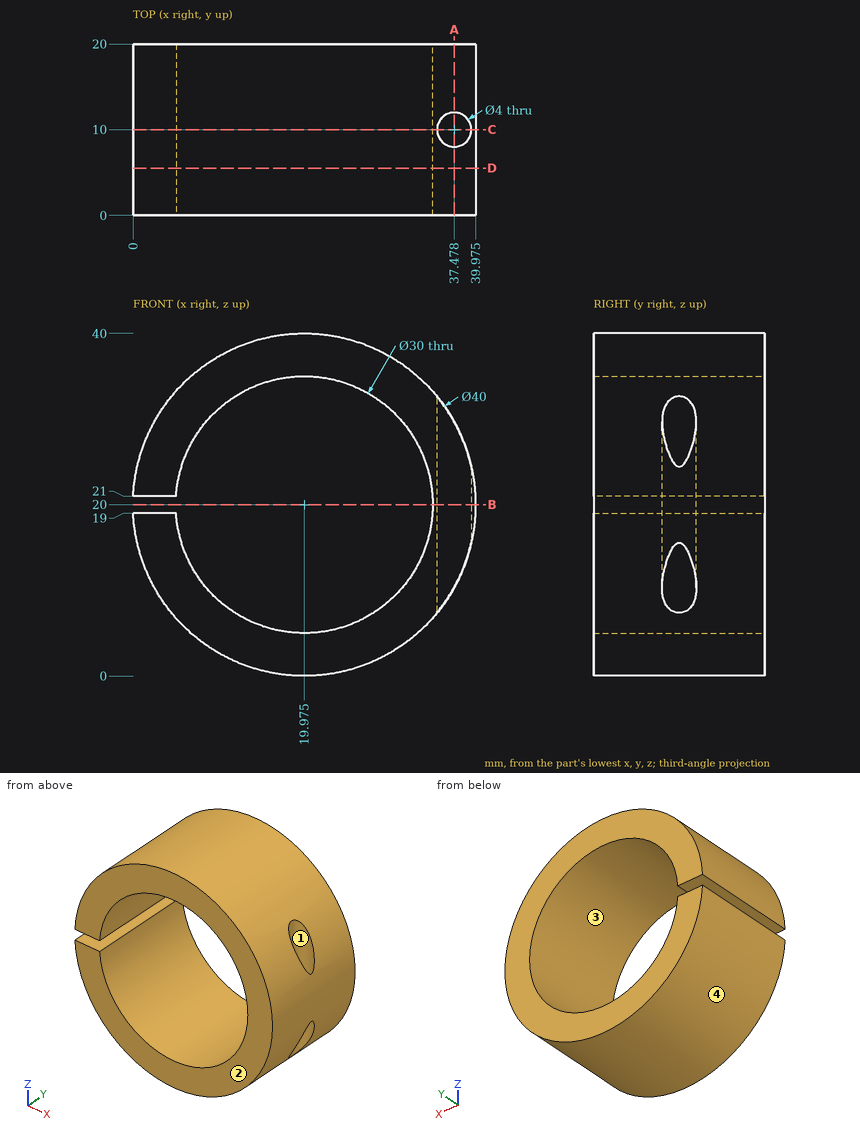
Input: dimensioned drawing with shaded views. Units: mm. Origin: part minimum x, y, z. Round coordinates to 2 decimals unless told otherwise and drop trailing zeros. Order: outer loops, then holes, each group sorted by start corner. A loop starts at its lowest first (then second) coordinate and runs counter-clockwise, first axis right, second up. Notation, with made-up numbers: (52, -31) - (76, -31) arc R32 ccw to (76, -3) - close; hole circle Ø11 at (38.5, 52). An arc over 180 degrees is marked (long way). Write item = value, one per line. Start each with the question number.
Q1. Cut plane B-B on z = 20. Return the cut outline in (x, y) (1 decimal).
Q2. Pin query (flat end, axial travel): pin 1 (6 mm diameter, centred on y = 6.5, z = 32, fed in from +X) (1 decimal); pin 2 (6 mm diameter, centred on y = 12.5, z = 30.5, fed in from -X) (1 decimal); pin 3 (8 mm diameter, centred on y = 2.5, z = 13.5, fed in from +X). Return the tip coordinate at first contact, or that it passes through.
Q3. Cut plane A-A on x = 37.5. Return the cut outline in (y, z), and give its area (3 significant figures).
Q4. Cut plane C-C on y = 10. Return the cut outline in (x, z) (1 decimal).
Q5. Cut plane D-D on y = 5.5. Return the cut outline in (x, z) (1 decimal), and give its area (3 significant figures).
Q6. Ray query, line 1 (Y direction, x = 37.5, z = 25.5); line 2 (Z direction, x = 20.5, y = 4); line 3 (Z direction, x = 11, y = 18.5) (1 decimal). Return the intervals inside material, ascending. Write a range as from..to.
Q7. Pull-direction query (X, two-part tool) for the marked faces 1, 2, 3 and 4; classes: +X half, -X half, draft (parallel to the pull), parting line (faces both ways), or undercut.
Outcome:
q1.outline = (35, 0) - (40, 0) - (40, 20) - (35, 20) - close; hole circle Ø4 at (37.5, 10)
q2.pin_1 = 37.8
q2.pin_2 = 1.4
q2.pin_3 = 39.82
q3.outline = (0, 10.36) - (8, 10.36) - (8, 29.64) - (0, 29.64) - close; (12, 10.36) - (20, 10.36) - (20, 29.64) - (12, 29.64) - close
q3.area = 308 mm^2
q4.outline = (0, 19) arc R20 ccw to (35.5, 7.4) - (35.5, 32.6) arc R20 ccw to (0, 21) - (5, 21) arc R15 cw (long way) to (5, 19) - close; (39.5, 15.6) arc R20 ccw to (39.5, 24.4) - close
q5.outline = (0, 19) arc R20 ccw (long way) to (0, 21) - (5, 21) arc R15 cw (long way) to (5, 19) - close
q5.area = 540 mm^2
q6.line_1 = 0..8, 12..20
q6.line_2 = 0.01..5.01, 34.99..39.99
q6.line_3 = 2.1..8, 32..37.9
q7.face_1 = undercut
q7.face_2 = draft
q7.face_3 = undercut
q7.face_4 = parting line
